Autodesk Inventor part; units mm, degrees
ref_plane "YZ Plane" through (0, 0, 0) normal (1, 0, 0) x (0, 1, 0)
ref_plane "XZ Plane" through (0, 0, 0) normal (0, 1, 0) x (-1, 0, 0)
ref_plane "XY Plane" through (0, 0, 0) normal (0, 0, 1) x (1, 0, 0)
sketch "Sketch2" plane through (0, 0, 0) normal (0, 0, 1) x (1, 0, 0)
  circle A0 centre (0, 0) radius 7.1 construction
  line L0 (-0.9625, 7.0345) -> (5.6108, 4.3508)
  line L1 (5.6108, 4.3508) -> (6.5733, -2.6837)
  line L2 (6.5733, -2.6837) -> (0.9625, -7.0345)
  line L3 (0.9625, -7.0345) -> (-5.6108, -4.3508)
  line L4 (-5.6108, -4.3508) -> (-6.5733, 2.6837)
  line L5 (-6.5733, 2.6837) -> (-0.9625, 7.0345)
  dimension "wheel_hexa_d" = 14.2
extrude "Extrusion1" add sketch "Sketch2" along normal blind 17
ref_plane "Work Plane1" through (0, 0, 2.89) normal (0, 0, -1) x (-1, 0, 0)
sketch "Sketch3" plane through (0, 0, 2.89) normal (0, 0, -1) x (-1, 0, 0)
  line L0 (6.5733, 2.6837) -> (0.9625, 7.0345)
  line L1 (-6.5733, -2.6837) -> (-0.9625, -7.0345)
  line L2 (0.9625, 7.0345) -> (6.5733, 2.6837) construction
  line L3 (3.7679, 4.8591) -> (-3.7679, -4.8591) construction
  line L4 (-0.9625, -7.0345) -> (-6.5733, -2.6837) construction
  circle A0 centre (0, 0) radius 3.715 construction
  line L5 (-3.4394, -1.4042) -> (-0.5036, -3.6807)
  line L6 (-0.5036, -3.6807) -> (2.9358, -2.2765)
  line L7 (2.9358, -2.2765) -> (3.4394, 1.4042)
  line L8 (3.4394, 1.4042) -> (0.5036, 3.6807)
  line L9 (0.5036, 3.6807) -> (-2.9358, 2.2765)
  line L10 (-2.9358, 2.2765) -> (-3.4394, -1.4042)
  dimension "d5" = 7.43
ref_plane "Work Plane2" through (-6.5733, 2.6837, 17) normal (-0.6128, 0.7902, 0) x (0.7902, 0.6128, 0)
sketch "Sketch4" plane through (-6.5733, 2.6837, 17) normal (-0.6128, 0.7902, 0) x (0.7902, 0.6128, 0)
  line L0 (7.1, 17) -> (7.1, 0) construction
  line L1 (0, 17) -> (0, 0) construction
  line L2 (0, 17) -> (7.1, 17) construction
  line L3 (7.1, 0) -> (0, 0) construction
  line L4 (6.37, 15.41) -> (0.73, 15.41)
  line L5 (0.73, 15.41) -> (0.73, 12.81)
  line L6 (0.73, 12.81) -> (6.37, 12.81)
  line L7 (6.37, 12.81) -> (6.37, 15.41)
  line L8 (-9.8809, 14.11) -> (16.8778, 14.11)
  line L9 (7.1, 14.11) -> (0, 14.11) construction
  line L10 (3.55, 15.41) -> (3.55, 12.81) construction
  point P0 (3.55, 17)
  point P1 (-0.165, 14)
  point P2 (-0.165, 10)
  point P3 (3.55, 14.11)
  point P4 (6.37, 14.11)
  dimension "d13" = 5.64
  dimension "d14" = 2.6
extrude "Extrusion3" cut sketch "Sketch4" against normal up to surface (12.2976 mm away)
ref_plane "Work Plane3" through (0, 0, 0) normal (0, 0, -1) x (-1, 0, 0)
sketch "Sketch5" plane through (0, 0, 0) normal (0, 0, -1) x (-1, 0, 0)
  circle A0 centre (0, 0) radius 1.6
  dimension "vis_d" = 3.2
extrude "Extrusion4" cut sketch "Sketch5" against normal blind 4.8
ref_plane "Work Plane4" through (0, 0, 17) normal (0, 0, 1) x (1, 0, 0)
sketch "Sketch6" plane through (0, 0, 17) normal (0, 0, 1) x (1, 0, 0)
  arc A0 (0.5392, 1.5064) -> (-1.5932, -0.1472) centre (0, 0) ccw construction
  line L0 (0.5392, 1.5064) -> (-1.5932, -0.1472)
  line L1 (-0.9625, 7.0345) -> (-6.5733, 2.6837) construction
  arc A1 (-1.5932, -0.1472) -> (0.5392, 1.5064) centre (0, 0) ccw
  line L2 (-2.7555, -1.0485) -> (-4.3487, 1.0062)
  line L3 (-4.3487, 1.0062) -> (0.1082, 4.4623)
  line L4 (0.1082, 4.4623) -> (1.7015, 2.4077)
  line L5 (1.7015, 2.4077) -> (-2.7555, -1.0485)
  line L6 (0, 0) -> (-3.7679, 4.8591) construction
  line L7 (-6.5733, 2.6837) -> (-0.9625, 7.0345) construction
  point P0 (-2.1202, 2.7343)
  dimension "d25" = 3.2
  dimension "d26" = 2.46
  dimension "petit_ecrou_cote" = 5.64
  dimension "petit_ecrou_depth" = 2.6
  dimension "d31" = 0
extrude "Extrusion5" cut sketch "Sketch6" against normal up to surface (12.81 mm away)
ref_plane "Work Plane5" through (-6.5733, 2.6837, 17) normal (-0.6128, 0.7902, 0) x (0.7902, 0.6128, 0)
sketch "Sketch7" plane through (-6.5733, 2.6837, 17) normal (-0.6128, 0.7902, 0) x (0.7902, 0.6128, 0)
  circle A0 centre (3.55, 3.82) radius 1.6
  line L0 (3.55, 3.82) -> (3.55, 0) construction
  line L1 (0.73, 0) -> (6.37, 0) construction
  point P0 (3.55, 17)
  dimension "d35" = 3.82
  dimension "d36" = 3.2
extrude "Extrusion6" cut sketch "Sketch7" against normal up to surface (5.2888 mm away)
sketch "Sketch8" plane through (0, 0, 10) normal (0, 0, -1) x (-1, 0, 0)
  circle A0 centre (0, 0) radius 9.2875
  dimension "d40" = 18.575
equation "\"big_hexa_depth\" = total_length"
equation "\"d5\" = ecrou_width"
equation "\"d13\" = petit_ecrou_cote"
equation "\"d14\" = petit_ecrou_depth"
equation "\"vis_d\" = vis_petit_ecrou_d"
equation "\"d25\" = vis_petit_ecrou_d"
equation "\"d32\" = petit_ecrou_hole_depth"
equation "\"d35\" = petit_ecrou_center_dist"
equation "\"d36\" = vis_petit_ecrou_d"
equation "\"d37\" = petit_ecrou_hole_depth"
equation "\"d40\" = 2.5 * ecrou_width"
equation "\"ecrou_dist\" = -vis_length_inside + 0.25 * petit_ecrou_hole_depth"
equation "\"ecrou_width\" = 7.43"
equation "\"ecrou_depth\" = 4"
equation "\"vis_petit_ecrou_d\" = 3.2"
equation "\"total_length\" = 17"
equation "\"d49\" = -vis_length_inside - petit_ecrou_cote"
properties part number "wheel_to_motor"
Work out the finished part from the listing and answer in its coordinate system (mm). A direction names the side the tool comes from. Round coordinates to 2 decimals unless told otherwise and drop trailing zeros. Write each loop counter-clockwise with the first axis right and the second up, starting at its lowest first coordinate (ties: lowest second). Pieces come first, ordered by that corner, then holes.
1) A cutting plane is placed at C-C on x = -3. Give the number of separate pieces and of enclosed holes in the cut face, and give its area (3 significant figures).
2) Determine the mould class of faces 4 (the face through (-3.23, 3.6, 14.74)), 5 (the face through (1.4, -1.5, 17)), 6 (the face through (-3.807, 4.829, 8.381)), 7 (the face through (-2.166, -0.592, 10.685)) for opening direction Y: pulls with the +Y half, pulls with the -Y half, needs draft (parallel to the pull), parting line crosses it, or undercut.
3) Consider probe 1 along Z at (x, y) = (1, 1.5); probe 2 along Z at (x, y) = (-1.25, 4); probe 3 along Z at (x, y) = (-2, 5). Determine where each line is inside the solid, lowest interval first.
4) A cutting plane is placed at D-D on y = -5.25. Determine the outline of the cut face in (x, z).
5) Flat-ended cylindrical pins translate along their axes: P1, Ø1.9, axis at x = 0, y = 0, coming from the +Z side; P2, Ø4, axis at x = -3, z = 2.5, coming from the +Y side; P3, Ø6, axis at y = 4, z = 11, coming from the +X side; P4, Ø2, axis at y = 4, z = 2, coming from the +X side. Find the tip coordinate at first contact, or state that the pin passes through.
6) Which of the six approach directions +Z, -Z, +X, -X, +Y, -Y give full straight-line access (tool end or side, diameter ignored) to faces 1 (the face through (0, -2, 4.19)), 2 (the face through (6.085, 0.883, 8.381)), 3 (the face through (1.128, 1.963, 10.685))?
7) A cutting plane is placed at A-A on x = -0.5. Determine the outline of the cut face in (y, z), and give its area (3 significant figures).
8) A cutting plane is placed at B-B on y = -2.25. Determine the outline of the cut face in (x, z), and give its area (3 significant figures).
Entries:
1. separate pieces: 3
1. enclosed holes: 0
1. area: 123 mm2
2. face 4: undercut
2. face 5: needs draft
2. face 6: pulls with the +Y half
2. face 7: undercut
3. probe 1: z = 0 to 1.59, 4.19 to 17
3. probe 2: z = 0 to 1.59, 4.19 to 12.53, 13.83 to 17
3. probe 3: z = 0 to 1.59, 4.19 to 12.58, 13.78 to 17
4. outline: (-3.41, 0) - (3.26, 0) - (3.26, 1.59) - (0.5, 1.59) - (0.5, 4.19) - (3.26, 4.19) - (3.26, 17) - (-3.41, 17) - close
5. P1: passes through
5. P2: stops at y = 7.01
5. P3: stops at x = 6.07
5. P4: stops at x = 5.8
6. face 1: none
6. face 2: +Z, -Z, +X, +Y
6. face 3: +Z
7. outline: (-6.44, 0) - (-1.52, 0) - (-1.52, 1.59) - (-3.96, 1.59) - (-3.96, 4.19) - (-1.52, 4.19) - (-1.52, 17) - (-6.44, 17) - close; (1.52, 0) - (6.85, 0) - (6.85, 17) - (3.99, 17) - (3.99, 4.19) - (5.25, 4.19) - (5.25, 1.59) - (1.52, 1.59) - close
7. area: 126 mm2
8. outline: (-5.9, 0) - (6.51, 0) - (6.51, 17) - (-5.9, 17) - close; hole (-1.82, 1.59) - (5.31, 1.59) - (5.31, 4.19) - (-1.82, 4.19) - close
8. area: 192 mm2
